```python
from build123d import *

# Parameters (mm, degrees)
SKETCH1_R           = 8.255
BOSS_EXTRUDE1_DEPTH = 2.3368
SKETCH2_R           = 2.38125
BOSS_EXTRUDE2_DEPTH = 14.605


with BuildPart() as part:
    # Sketch1 → Boss-Extrude1 (new body)
    with BuildSketch(Plane.XY):
        Circle(SKETCH1_R)
    extrude(amount=BOSS_EXTRUDE1_DEPTH)

    # Sketch2 → Boss-Extrude2 (add)
    with BuildSketch(Plane.XY):
        Circle(SKETCH2_R)
    extrude(amount=-BOSS_EXTRUDE2_DEPTH)

    # Sketch3 → Cut-Revolve1 (revolve, cut)
    with BuildSketch(Plane(origin=(0, 0, 0), x_dir=(1, 0, 0), z_dir=(0, 1, 0))):
        with BuildLine():
            ThreePointArc((1.4478, -2.3368), (4.989096566, -1.838155581), (8.255, -0.381))
            Line((8.255, -0.381), (8.255, -2.3368))
            Line((8.255, -2.3368), (1.4478, -2.3368))
        make_face()
    revolve(axis=Axis((0, 0, 2.3368), (0, 0, -1)), mode=Mode.SUBTRACT)


solid = part.part
```
Verification items for the finished model (mm, model axes). A direction names the side the tool comes from. Coordinates: 2 decimals unless noted, no trailing zeros. Loops run counter-clockwise (first coordinate to the right, second up) from the corner with the lowest first, then second, coordinate; pieces in that order, holes last. Notation, with made-up numbers: (-23, 82) - (-5, 82) arc R11 ccw to (-5, 86) - close; hole circle Ø1 at (-26, 54.25). An arc over 180 degrees is marked (long way). Answer as a JSON object with one key per item and string values.
(1) Scan lines: line 1 along Z through (x, y) = (-1.75, -4); line 2 along Z through (x, y) = (0.5, 2.5); line 3 along X through (y, z) = (-0.25, -1.75). Record each from-to range of solid material in increasing order.
Response:
{"line 1": "z = 0 to 2", "line 2": "z = 0 to 2.29", "line 3": "x = -2.37 to 2.37"}
(2) Go/stop test with flat-tipped pins: pin 1 Ø2 at (y, z) = (2, -4.5) entering from -X; pin 2 Ø1.5 at (x, y) = (5, -2.5) entering from +Z; pin 3 Ø8 at (x, z) = (1.5, -6) entering from -Y; pin 4 Ø2 at (x, z) = (-3.5, -1.5) entering from +Y. Record where each tip stops, or that it passes through.
Response:
{"pin 1": "stops at x = -2.16", "pin 2": "stops at z = 1.88", "pin 3": "stops at y = -2.38", "pin 4": "passes through"}
(3) Cross-section at A-A, the plane z = -5.5. Record the boundary of the cut face in (x, y).
Response:
{"outline": "circle Ø4.76 at (0, 0)"}
(4) Access from +Z, -Z, +X, -X, +Y, -Y to the whole of each face (thin tool, end or side, straight path). Record for faces 1 (the flat face through (0, 0, 2.337)), 2 (the cylindrical face through (-1.89, -1.45, -7.2)).
Response:
{"face 1": "+Z, +X, -X, +Y, -Y", "face 2": "-Z"}
